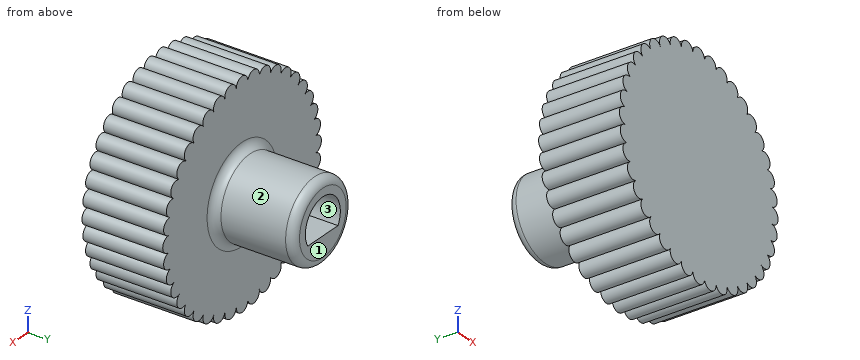
```python
from build123d import *

# Parameters (mm, degrees)
BOSS_EXTRUDE2_DEPTH = 10
SKETCH2_R           = 5
BOSS_EXTRUDE3_DEPTH = 10
FILLET5_R           = 1
FILLET7_R           = 1


with BuildPart() as part:
    # Sketch1 → Boss-Extrude2 (new body)
    with BuildSketch(Plane(origin=(0, 0, 0), x_dir=(1, 0, 0), z_dir=(0, 1, 0))):
        with BuildLine():
            ThreePointArc((0.986735573, 12.537664208), (0, 13.605108736), (-0.986735573, 12.537664208))
            ThreePointArc((-0.986735573, 12.537664208), (-2.128307907, 13.437607271), (-2.935910014, 12.228945305))
            ThreePointArc((-2.935910014, 12.228945305), (-4.20420981, 12.939227319), (-4.812792606, 11.619109183))
            ThreePointArc((-4.812792606, 11.619109183), (-6.176590114, 12.122240646), (-6.571168272, 10.723172031))
            ThreePointArc((-6.571168272, 10.723172031), (-7.996882271, 11.006764178), (-8.167739967, 9.563194796))
            ThreePointArc((-8.167739967, 9.563194796), (-9.620264646, 9.620264646), (-9.563194796, 8.167739967))
            ThreePointArc((-9.563194796, 8.167739967), (-11.006764178, 7.996882271), (-10.723172031, 6.571168272))
            ThreePointArc((-10.723172031, 6.571168272), (-12.122240646, 6.176590114), (-11.619109183, 4.812792606))
            ThreePointArc((-11.619109183, 4.812792606), (-12.939227319, 4.20420981), (-12.228945305, 2.935910014))
            ThreePointArc((-12.228945305, 2.935910014), (-13.437607271, 2.128307907), (-12.537664208, 0.986735573))
            ThreePointArc((-12.537664208, 0.986735573), (-13.605108736, 0), (-12.537664208, -0.986735573))
            ThreePointArc((-12.537664208, -0.986735573), (-13.437607271, -2.128307907), (-12.228945305, -2.935910014))
            ThreePointArc((-12.228945305, -2.935910014), (-12.939227319, -4.20420981), (-11.619109183, -4.812792606))
            ThreePointArc((-11.619109183, -4.812792606), (-12.122240646, -6.176590114), (-10.723172031, -6.571168272))
            ThreePointArc((-10.723172031, -6.571168272), (-11.006764178, -7.996882271), (-9.563194796, -8.167739967))
            ThreePointArc((-9.563194796, -8.167739967), (-9.620264646, -9.620264646), (-8.167739967, -9.563194796))
            ThreePointArc((-8.167739967, -9.563194796), (-7.996882271, -11.006764178), (-6.571168272, -10.723172031))
            ThreePointArc((-6.571168272, -10.723172031), (-6.176590114, -12.122240646), (-4.812792606, -11.619109183))
            ThreePointArc((-4.812792606, -11.619109183), (-4.20420981, -12.939227319), (-2.935910014, -12.228945305))
            ThreePointArc((-2.935910014, -12.228945305), (-2.128307907, -13.437607271), (-0.986735573, -12.537664208))
            ThreePointArc((-0.986735573, -12.537664208), (0, -13.605108736), (0.986735573, -12.537664208))
            ThreePointArc((0.986735573, -12.537664208), (2.128307907, -13.437607271), (2.935910014, -12.228945305))
            ThreePointArc((2.935910014, -12.228945305), (4.20420981, -12.939227319), (4.812792606, -11.619109183))
            ThreePointArc((4.812792606, -11.619109183), (6.176590114, -12.122240646), (6.571168272, -10.723172031))
            ThreePointArc((6.571168272, -10.723172031), (7.996882271, -11.006764178), (8.167739967, -9.563194796))
            ThreePointArc((8.167739967, -9.563194796), (9.620264646, -9.620264646), (9.563194796, -8.167739967))
            ThreePointArc((9.563194796, -8.167739967), (11.006764178, -7.996882271), (10.723172031, -6.571168272))
            ThreePointArc((10.723172031, -6.571168272), (12.122240646, -6.176590114), (11.619109183, -4.812792606))
            ThreePointArc((11.619109183, -4.812792606), (12.939227319, -4.20420981), (12.228945305, -2.935910014))
            ThreePointArc((12.228945305, -2.935910014), (13.437607271, -2.128307907), (12.537664208, -0.986735573))
            ThreePointArc((12.537664208, -0.986735573), (13.605108736, 0), (12.537664208, 0.986735573))
            ThreePointArc((12.537664208, 0.986735573), (13.437607271, 2.128307907), (12.228945305, 2.935910014))
            ThreePointArc((12.228945305, 2.935910014), (12.939227319, 4.20420981), (11.619109183, 4.812792606))
            ThreePointArc((11.619109183, 4.812792606), (12.122240646, 6.176590114), (10.723172031, 6.571168272))
            ThreePointArc((10.723172031, 6.571168272), (11.006764178, 7.996882271), (9.563194796, 8.167739967))
            ThreePointArc((9.563194796, 8.167739967), (9.620264646, 9.620264646), (8.167739967, 9.563194796))
            ThreePointArc((8.167739967, 9.563194796), (7.996882271, 11.006764178), (6.571168272, 10.723172031))
            ThreePointArc((6.571168272, 10.723172031), (6.176590114, 12.122240646), (4.812792606, 11.619109183))
            ThreePointArc((4.812792606, 11.619109183), (4.20420981, 12.939227319), (2.935910014, 12.228945305))
            ThreePointArc((2.935910014, 12.228945305), (2.128307907, 13.437607271), (0.986735573, 12.537664208))
        make_face()
    extrude(amount=BOSS_EXTRUDE2_DEPTH)

    # Sketch2 → Boss-Extrude3 (add)
    with BuildSketch(Plane(origin=(0, 10, 0), x_dir=(1, 0, 0), z_dir=(0, 1, 0))):
        with Locations(Location((0, 0, 0), (0, 0, 270))):
            Circle(SKETCH2_R)
        with BuildLine():
            Line((-2.598076211, 1.5), (2.598076211, 1.5))
            ThreePointArc((2.598076211, 1.5), (0, -3), (-2.598076211, 1.5))
        make_face(mode=Mode.SUBTRACT)
    extrude(amount=BOSS_EXTRUDE3_DEPTH)

    # Fillet5
    fillet5_edges = [part.edges().sort_by_distance(p)[0] for p in [
        (0, 20, -5),
    ]]
    fillet(fillet5_edges, radius=FILLET5_R)

    # Fillet7
    fillet7_edges = [part.edges().sort_by_distance(p)[0] for p in [
        (0, 10, -5),
    ]]
    fillet(fillet7_edges, radius=FILLET7_R)


solid = part.part
```
For this review, take the finished solid that the model builds, in its own axes (mm). Face numbers are marked on the shaded views. Give positions to 0.01 mm unless a question says otherwise; leave off trailing zeros. Write each loop counter-clockwise with the first axis right and the second up, starting at its lowest first coordinate (ties: lowest second). Pieces come first, ordered by that corner, then holes.
Item 1: Insertion check: P1, Ø12, axis at y = 10.5, z = 2, coming from the -X side; P2, Ø4, axis at y = 6, z = 4, coming from the -X side; P3, Ø1.5, axis at x = -2, y = 7.5, coming from the +Z side; P4, Ø4, axis at x = 5.5, y = 4, coming from the +Z side. Each pin has a flat end and moves straight along its axis. Give the tip position at first contact, or say it passes through.
Item 2: The part is to be moulded in two halves that separate along X. For the marked faces 1, 2 and 3, say which applies: +X half, -X half, draft (parallel to the pull), parting line (faces both ways), or undercut.
Item 3: Take a section at B-B (z = 0). Give the boundary of the cut face in (x, y), and give its area (3 significant figures).
Item 4: Wall thickness on probe 1 along X at (y, z) = (17.5, 0); probe 2 along Y at (x, z) = (-3.75, -12.5); probe 3 along X at (y, z) = (17, 4.25): over which ranges is each line inside the solid? List them lowest first.
Item 5: Take a section at A-A (x = 0). Give the boundary of the cut face in (y, z), and give its area (3 significant figures).
Item 6: Take a section at C-C (y = 14). Give the boundary of the cut face in (x, z), and give its area (3 significant figures).
Established:
1. P1: stops at x = -13.61
1. P2: stops at x = -13.45
1. P3: stops at z = 13.45
1. P4: stops at z = 12.99
2. face 1: draft
2. face 2: parting line
2. face 3: undercut
3. outline: (-13.61, 0) - (13.61, 0) - (13.61, 10) - (6, 10) arc R1 cw to (5, 11) - (5, 19) arc R1 ccw to (4, 20) - (3, 20) - (3, 10) - (-3, 10) - (-3, 20) - (-4, 20) arc R1 ccw to (-5, 19) - (-5, 11) arc R1 cw to (-6, 10) - (-13.61, 10) - close
3. area: 312 mm2
4. probe 1: x = -5 to -3, 3 to 5
4. probe 2: y = 0 to 10
4. probe 3: x = -2.63 to 2.63
5. outline: (0, -13.61) - (10, -13.61) - (10, -6) arc R1 cw to (11, -5) - (19, -5) arc R1 ccw to (20, -4) - (20, -1.5) - (10, -1.5) - (10, 3) - (20, 3) - (20, 4) arc R1 ccw to (19, 5) - (11, 5) arc R1 cw to (10, 6) - (10, 13.61) - (0, 13.61) - close
5. area: 327 mm2
6. outline: circle Ø10 at (0, 0); hole (-2.6, -1.5) - (2.6, -1.5) arc R3 ccw (long way) to start
6. area: 55.8 mm2
